```python
from build123d import *

# Parameters (mm, degrees)
F0_W      = 130
F0_H      = 150
F1_DEPTH  = 51
F2_W      = 128
F2_H      = 49
F3_DEPTH  = 130.001
F4_W      = 90
F4_H      = 35
F5_DEPTH  = 3
F6_R      = 5
F7_R      = 5
F8_R      = 2
F9_R      = 2
F11_DEPTH = 1
F12_W     = 40
F12_H     = 25
F13_DEPTH = 1
F15_DEPTH = 2
F16_SIZE  = 1
F18_DEPTH = 2


with BuildPart() as f1:
    # F0 (on Top) → F1 (new body)
    with BuildSketch(Plane.XY):
        Rectangle(F0_W, F0_H)
    extrude(amount=F1_DEPTH)

    # F2 (on face) → F3 (cut, through all)
    with BuildSketch(Plane.YZ.offset(65)):
        with Locations((11, 24.5)):
            Rectangle(F2_W, F2_H)
    extrude(amount=-F3_DEPTH, mode=Mode.SUBTRACT)

    # F4 (on face) → F5 (cut)
    with BuildSketch(Plane.XZ.offset(75)):
        with Locations((0, 25.5)):
            Rectangle(F4_W, F4_H)
    extrude(amount=-F5_DEPTH, mode=Mode.SUBTRACT)

    # F6
    f6_edges = [f1.edges().sort_by_distance(p)[0] for p in [
        (-45, -73.5, 43),
    ]]
    fillet(f6_edges, radius=F6_R)

    # F7
    f7_edges = [f1.edges().sort_by_distance(p)[0] for p in [
        (45, -73.5, 43),
        (45, -73.5, 8),
        (-45, -73.5, 8),
    ]]
    fillet(f7_edges, radius=F7_R)

    # F8
    f8_edges = [f1.edges().sort_by_distance(p)[0] for p in [
        (0, -75, 0),
    ]]
    fillet(f8_edges, radius=F8_R)

    # F9
    f9_edges = [f1.edges().sort_by_distance(p)[0] for p in [
        (0, -75, 51),
    ]]
    fillet(f9_edges, radius=F9_R)

    # F10 (on face) → F11 (join)
    with BuildSketch(Plane(origin=(0, -53, 0), x_dir=(-1, 0, 0), z_dir=(0, 1, 0))):
        with BuildLine():
            Line((-57, 39.1), (-57, 17.1))
            ThreePointArc((-57, 17.1), (-56.5606601718, 16.0393398282), (-55.5, 15.6))
            ThreePointArc((-55.5, 15.6), (-54.4393398282, 16.0393398282), (-54, 17.1))
            Line((-54, 17.1), (-54, 39.1))
            ThreePointArc((-54, 39.1), (-54.4393398282, 40.1606601718), (-55.5, 40.6))
            ThreePointArc((-55.5, 40.6), (-56.5606601718, 40.1606601718), (-57, 39.1))
        make_face()
    extrude(amount=F11_DEPTH)

    # F12 (on face) → F13 (cut)
    with BuildSketch(Plane(origin=(0, -53, 0), x_dir=(-1, 0, 0), z_dir=(0, 1, 0))):
        with Locations((-11, 35.5)):
            Rectangle(F12_W, F12_H)
    extrude(amount=-F13_DEPTH, mode=Mode.SUBTRACT)

    # F14 (on face) → F15 (cut)
    with BuildSketch(Plane(origin=(0, -53, 0), x_dir=(-1, 0, 0), z_dir=(0, 1, 0))):
        with BuildLine():
            Line((-24, 16), (-24, 6))
            Line((-24, 6), (-5, 6))
            ThreePointArc((-5, 6), (-1.4644660941, 7.4644660941), (0, 11))
            ThreePointArc((0, 11), (-1.4644660941, 14.5355339059), (-5, 16))
            Line((-5, 16), (-24, 16))
        make_face()
        with BuildLine():
            ThreePointArc((-24, 16), (-27.5355339059, 14.5355339059), (-29, 11))
            ThreePointArc((-29, 11), (-27.5355339059, 7.4644660941), (-24, 6))
            Line((-24, 6), (-24, 16))
        make_face()
    extrude(amount=-F15_DEPTH, mode=Mode.SUBTRACT)

    # F16
    f16_edges = [f1.edges().sort_by_distance(p)[0] for p in [
        (29, -55, 11),
        (14.5, -55, 16),
        (0, -55, 11),
        (14.5, -55, 6),
    ]]
    chamfer(f16_edges, length=F16_SIZE)

    # F17 (on face) → F18 (join)
    with BuildSketch(Plane(origin=(0, -55, 0), x_dir=(-1, 0, 0), z_dir=(0, 1, 0))):
        with BuildLine():
            Line((-27, 11), (-24, 11))
            Line((-24, 11), (-17, 11))
            ThreePointArc((-17, 11), (-17.4393398282, 12.0606601718), (-18.5, 12.5))
            Line((-18.5, 12.5), (-25.5, 12.5))
            ThreePointArc((-25.5, 12.5), (-26.5606601718, 12.0606601718), (-27, 11))
        make_face()
        with BuildLine():
            Line((-17, 11), (-24, 11))
            Line((-24, 11), (-27, 11))
            ThreePointArc((-27, 11), (-26.5606601718, 9.9393398282), (-25.5, 9.5))
            Line((-25.5, 9.5), (-18.5, 9.5))
            ThreePointArc((-18.5, 9.5), (-17.4393398282, 9.9393398282), (-17, 11))
        make_face()
        with BuildLine():
            ThreePointArc((-10.5000000544, 12.4815619213), (-11.5606602262, 12.042222093), (-12.0000000544, 10.9815619213))
            ThreePointArc((-12.0000000544, 10.9815619213), (-11.5606602262, 9.9209017495), (-10.5000000544, 9.4815619213))
            Line((-10.5000000544, 9.4815619213), (-3.5000000544, 9.4815619213))
            ThreePointArc((-3.5000000544, 9.4815619213), (-2.4393398827, 9.9209017495), (-2.0000000544, 10.9815619213))
            ThreePointArc((-2.0000000544, 10.9815619213), (-2.4393398827, 12.042222093), (-3.5000000544, 12.4815619213))
            Line((-3.5000000544, 12.4815619213), (-10.5000000544, 12.4815619213))
        make_face()
    extrude(amount=F18_DEPTH)


solid = f1.part
```
Here's how the part is built. I have some questions about the finished solid (model axes, mm). A direction names the side the tool comes from. Coordinates: 2 decimals unless noted, no trailing zeros. Order: outer loops, then holes, each group sorted by start corner. A loop starts at its lowest first (then second) coordinate and runs counter-clockwise, first axis right, second up. Notation, with made-up numbers: (49.5, 11.5) - (83.5, 11.5) arc R32 ccw to (83.5, 43.5) - close; hole circle Ø1 at (-20.5, 18). An arc over 180 degrees is marked (long way). One line per question, with ' | ' between items. Start each with the question number.
1. Which directions (+Z, -Z, +X, -X, +Y, -Y) give clear straight access to the entire face, cutting with the end or side of a thin tool? Please do faces 1 (the flat face through (-1, -75, 46)), 2 (the flat face through (15, -55, 11)), 3 (the cylindrical face through (-44, -73, 10)).
2. If we section it at D-D (x = -55.5): Write out the boundary of the cut face in (y, z).
3. If we section it at A-A (z = 30): Write out the boundary of the cut face in (x, y), and give its area (3 significant figures).
4. If we section it at B-B (x = 35): Write out the boundary of the cut face in (y, z), and give its area (3 significant figures).
5. Please list where these lines run through material, in increasing order: line 1 along Z through (x, y) = (-27.5, -28); line 2 along Y through (x, z) = (-31, 39.5); line 3 along Y through (x, z) = (-46.5, 34). Write a range as [from, to].
6. If we section it at C-C (y = 11.5): Write out the boundary of the cut face in (x, z), and give its area (3 significant figures).
7. If we mould it in two halves opening along Z, with no side actions, what happens to faces 4 (the flat face through (-1, 2, 51)), 5 (the cylindrical face through (43, -73, 42)), 6 (the flat face through (-65, -56, 29))? For each: released by +Z, released by -Z, zero draft, split by the parting line, or undercut.
8. I'm going to push flat-ended pins straight in: pin 1 Ø1.5 at (x, z) = (55, 28) entering from +Y; pin 2 Ø1.1 at (y, z) = (-52.5, 31.5) entering from +X; pin 3 Ø1.5 at (x, y) = (-20, -50.5) entering from -Z; pin 4 Ø0.5 at (y, z) = (-52.5, 32) entering from -X. Where does each tip first touch, or does it pass through?
Model answer:
1) face 1: +Z, -Z, +X, -X, -Y | face 2: +Y | face 3: -Y
2) outline: (-75, 2) arc R2 ccw to (-73, 0) - (-53, 0) - (-53, 49) - (75, 49) - (75, 51) - (-73, 51) arc R2 ccw to (-75, 49) - close
3) outline: (-65, -75) - (-45, -75) - (-45, -72) - (45, -72) - (45, -75) - (65, -75) - (65, -53) - (57, -53) - (57, -52) - (54, -52) - (54, -53) - (31, -53) - (31, -54) - (-9, -54) - (-9, -53) - (-65, -53) - close | area: 2,550 mm²
4) outline: (-75, 2) arc R2 ccw to (-73, 0) - (-53, 0) - (-53, 49) - (75, 49) - (75, 51) - (-73, 51) arc R2 ccw to (-75, 49) - (-75, 43) - (-72, 43) - (-72, 8) - (-75, 8) - close | area: 1,270 mm²
5) line 1: z = [49, 51] | line 2: y = [-72, -53] | line 3: y = [-75, -53]
6) outline: (-65, 49) - (65, 49) - (65, 51) - (-65, 51) - close | area: 260 mm²
7) face 4: released by +Z | face 5: undercut | face 6: zero draft
8) pin 1: stops at y = -52 | pin 2: stops at x = 65 | pin 3: stops at z = 49 | pin 4: stops at x = 54
